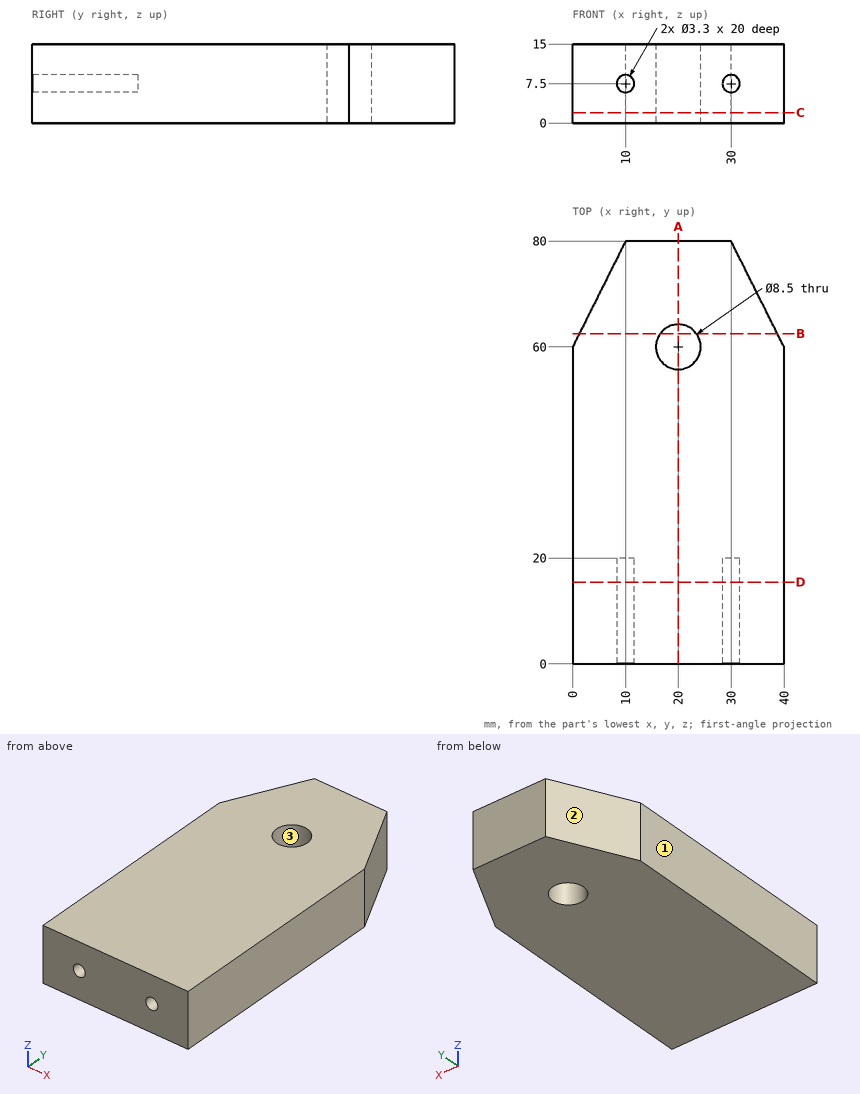
Geometry check sheet. Reference: drawing and pictorial views, mm from the part's lowest x, y, z. Round coordinates to 2 decimals unless told otherwise and drop trailing zeros. Loops run counter-clockwise (first coordinate to the right, second up) from the corner with the lowest first, then second, coordinate; pieces in that order, holes last. Notation, with made-up numbers: M 77,60.25 L 90,60.25 A8 ccw 90,66.25 Z; hole C -30.5,81.25 d10. An arc over 180 degrees is marked long. One line per item, written item: value.
(1) Sectioned sample at D-D, the plane y = 15.5. Record the cut outline in (x, z), then the cut area to 3 significant figures.
Computed values:
outline: M 0,0 L 40,0 L 40,15 L 0,15 Z; hole C 10,7.5 d3.3; hole C 30,7.5 d3.3
area: 583 mm^2
(2) Sectioned sample at B-B, the plane y = 62.5. Record the cut outline in (x, z), then the cut area to 3 significant figures.
Computed values:
outline: M 1.25,0 L 16.56,0 L 16.56,15 L 1.25,15 Z; M 23.44,0 L 38.75,0 L 38.75,15 L 23.44,15 Z
area: 459 mm^2
(3) Sectioned sample at C-C, the plane z = 2. Record the cut outline in (x, y), then the cut area to 3 significant figures.
Computed values:
outline: M 0,0 L 40,0 L 40,60 L 30,80 L 10,80 L 0,60 Z; hole C 20,60 d8.5
area: 2,940 mm^2
(4) Thickness scan on line 1 (Z direction, x = 30, y = 11); line 2 (Y direction, x = 20, z = 11.25); line 3 (Y direction, x = 17, z = 7.5). Record the ranges inside material, lowest first.
Computed values:
line 1: z = 0 to 5.85, 9.15 to 15
line 2: y = 0 to 55.75, 64.25 to 80
line 3: y = 0 to 56.99, 63.01 to 80
(5) Sectioned sample at A-A, the plane x = 20. Record the cut outline in (y, z), then the cut area to 3 significant figures.
Computed values:
outline: M 0,0 L 55.75,0 L 55.75,15 L 0,15 Z; M 64.25,0 L 80,0 L 80,15 L 64.25,15 Z
area: 1,070 mm^2
(6) Release check for a two-part mould opening along Y. For the marked faces 1, 2 and 3 record: +Y half, -Y half, draft (parallel to the pull), parting line (faces both ways), or undercut.
Computed values:
face 1: draft
face 2: +Y half
face 3: undercut
(7) Depth check by flat-ended pin: pin 1 Ø1 at (x, z) = (9, 8) entering from +Y; pin 2 Ø1 at (x, z) = (29.5, 7.5) entering from -Y; pin 3 Ø1.5 at (y, z) = (67.5, 13.5) entering from -X (3 decimals). Enter the tip coordinate at first touch or a pass-through.
Computed values:
pin 1: stops at y = 79
pin 2: stops at y = 20
pin 3: stops at x = 3.375
